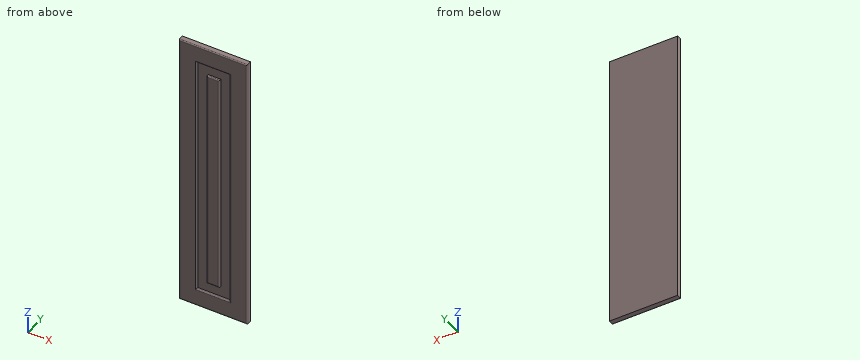
```python
from build123d import *

# Parameters (mm, degrees)
F0_W      = 44.656470418
F0_H      = 33.8078811765
F1_DEPTH  = 16
F2_DEPTH  = 796
F3_DEPTH  = 196
F4_W      = 68.9578056335
F4_H      = 493.6993122101
F5_DEPTH  = 7
F6_DEPTH  = 9.7
F7_DEPTH  = 99.33
F8_DEPTH  = 99.33
F9_DEPTH  = 17.34
F10_DEPTH = 102.97
F11_W     = 35.2807044983
F11_H     = 492.0964837074
F12_DEPTH = 7
F13_DEPTH = 37.27
F14_DEPTH = 6.58
F15_DEPTH = 106.63
F16_DEPTH = 5.87
F17_R     = 3


with BuildPart() as f1:
    # F0 (on Front) → F1 (new body)
    with BuildSketch(Plane.XZ):
        with Locations((22.328235209, 16.9039405882)):
            Rectangle(F0_W, F0_H)
    extrude(amount=F1_DEPTH)

    # F2 (add): a face of the model
    f2_faces = [f1.faces().sort_by_distance(p)[0] for p in [
        (22.328235209, -8, 0),
    ]]
    extrude(f2_faces, amount=-F2_DEPTH)

    # F3 (add): a face of the model
    f3_faces = [f1.faces().sort_by_distance(p)[0] for p in [
        (0, -8, 398),
    ]]
    extrude(f3_faces, amount=-F3_DEPTH)

    # F4 (on face) → F5 (cut)
    with BuildSketch(Plane.XZ.offset(16)):
        with Locations((94.1769480705, 399.8196721077)):
            Rectangle(F4_W, F4_H)
    extrude(amount=-F5_DEPTH, mode=Mode.SUBTRACT)

    # F6 (cut): a face of the model
    f6_faces = [f1.faces().sort_by_distance(p)[0] for p in [
        (59.6980452538, -12.5, 399.8196721077),
    ]]
    extrude(f6_faces, amount=-F6_DEPTH, mode=Mode.SUBTRACT)

    # F7 (add): a face of the model
    f7_faces = [f1.faces().sort_by_distance(p)[0] for p in [
        (89.3269480705, -12.5, 646.6693282127),
    ]]
    extrude(f7_faces, amount=-F7_DEPTH)

    # F8 (cut): a face of the model
    f8_faces = [f1.faces().sort_by_distance(p)[0] for p in [
        (89.3269480705, -12.5, 646.6693282127),
    ]]
    extrude(f8_faces, amount=-F8_DEPTH, mode=Mode.SUBTRACT)

    # F9 (cut): a face of the model
    f9_faces = [f1.faces().sort_by_distance(p)[0] for p in [
        (128.6558508873, -12.5, 449.4846721077),
    ]]
    extrude(f9_faces, amount=-F9_DEPTH, mode=Mode.SUBTRACT)

    # F10 (cut): a face of the model
    f10_faces = [f1.faces().sort_by_distance(p)[0] for p in [
        (97.9969480705, -12.5, 152.9700160027),
    ]]
    extrude(f10_faces, amount=-F10_DEPTH, mode=Mode.SUBTRACT)

    # F11 (on face) → F12 (join)
    with BuildSketch(Plane.XZ.offset(9)):
        with Locations((91.7714834213, 432.6795041561)):
            Rectangle(F11_W, F11_H)
    extrude(amount=F12_DEPTH)

    # F13 (add): a face of the model
    f13_faces = [f1.faces().sort_by_distance(p)[0] for p in [
        (91.7714834213, -12.5, 678.7277460098),
    ]]
    extrude(f13_faces, amount=F13_DEPTH)

    # F14 (add): a face of the model
    f14_faces = [f1.faces().sort_by_distance(p)[0] for p in [
        (109.4118356705, -12.5, 451.3145041561),
    ]]
    extrude(f14_faces, amount=F14_DEPTH)

    # F15 (add): a face of the model
    f15_faces = [f1.faces().sort_by_distance(p)[0] for p in [
        (95.0614834213, -12.5, 186.6312623024),
    ]]
    extrude(f15_faces, amount=F15_DEPTH)

    # F16 (cut): a face of the model
    f16_faces = [f1.faces().sort_by_distance(p)[0] for p in [
        (74.1311311722, -12.5, 397.9995041561),
    ]]
    extrude(f16_faces, amount=-F16_DEPTH, mode=Mode.SUBTRACT)

    # F17
    f17_edges = [f1.edges().sort_by_distance(p)[0] for p in [
        (0, -16, 398),
        (98, -16, 0),
        (196, -16, 398),
        (98, -16, 796),
        (145.995851, -16, 397.999672),
        (97.996948, -16, 50.000016),
        (49.998045, -16, 397.999672),
        (97.996948, -16, 745.999328),
        (97.996483, -16, 715.997746),
        (115.991836, -16, 397.999504),
        (97.996483, -16, 80.001262),
        (80.001131, -16, 397.999504),
    ]]
    fillet(f17_edges, radius=F17_R)


solid = f1.part
```
Can you work these out from the model? Positions are in its coordinate system, mm. Give positions to 0.01 mm unless a question says otherwise; leave off trailing zeros. Order: outer loops, then holes, each group sorted by start corner. A loop starts at its lowest first (then second) coordinate and runs counter-clockwise, first axis right, second up. Notation, with made-up numbers: (40.5, 38) - (81.5, 38) arc R18 ccw to (81.5, 65) - close; hole circle Ø8 at (53, -23). An arc over 180 degrees is marked (long way). Use a Markdown table: item, result. Add a question column.
Q1. If we section it at D-D on x = 92.5: Write out the boundary of the cut face in (y, z), plus the area to 3 significant figures.
Q2. If we section it at B-B on z = 734: Write out the boundary of the cut face in (x, y), plus the area to 3 significant figures.
Q3. Please list where these lines run through material, in increasing order: line 1 along X through (y, z) = (-11.75, 486.5); line 2 along Z through (x, y) = (113.5, -13.25); line 3 along Z through (x, y) = (128, -12.75).
Q4. If we section it at C-C on z = 562: Write out the boundary of the cut face in (x, y).
Q5. If we section it at A-A on x = 60: Write out the boundary of the cut face in (y, z).
Answers follow:
| question | item | result |
|---|---|---|
| 1 | outline | (-16, 3) arc R3 ccw to (-13, 0) - (0, 0) - (0, 796) - (-13, 796) arc R3 ccw to (-16, 793) - (-16, 749) arc R3 ccw to (-13, 746) - (-9, 746) - (-9, 716) - (-13, 716) arc R3 ccw to (-16, 713) - (-16, 83) arc R3 ccw to (-13, 80) - (-9, 80) - (-9, 50) - (-13, 50) arc R3 ccw to (-16, 47) - close |
| 1 | area | 12,300 mm^2 |
| 2 | outline | (0, -13) arc R3 ccw to (3, -16) - (47, -16) arc R3 ccw to (50, -13) - (50, -9) - (146, -9) - (146, -13) arc R3 ccw to (149, -16) - (193, -16) arc R3 ccw to (196, -13) - (196, 0) - (0, 0) - close |
| 2 | area | 2,460 mm^2 |
| 3 | line 1 | x = 0 to 50, 80 to 115.99, 146 to 196 |
| 3 | line 2 | z = 0.01 to 49.99, 80.01 to 715.99, 746.01 to 795.99 |
| 3 | line 3 | z = 0 to 50, 746 to 796 |
| 4 | outline | (0, -13) arc R3 ccw to (3, -16) - (47, -16) arc R3 ccw to (50, -13) - (50, -9) - (80, -9) - (80, -13) arc R3 ccw to (83, -16) - (112.99, -16) arc R3 ccw to (115.99, -13) - (115.99, -9) - (146, -9) - (146, -13) arc R3 ccw to (149, -16) - (193, -16) arc R3 ccw to (196, -13) - (196, 0) - (0, 0) - close |
| 5 | outline | (-16, 3) arc R3 ccw to (-13, 0) - (0, 0) - (0, 796) - (-13, 796) arc R3 ccw to (-16, 793) - (-16, 749) arc R3 ccw to (-13, 746) - (-9, 746) - (-9, 50) - (-13, 50) arc R3 ccw to (-16, 47) - close |
